The listing builds one solid part. Answer for the finished solid, in the listing's coordinates (mm). Face numbers are marked on the shaded views. A direction names the side the tool comes from. Round coordinates to 2 decimals unless told otherwise and drop trailing zeros. Order: outer loops, then holes, each group sorted by start corner. A loop starts at its lowest first (then second) coordinate and runs counter-clockwise, first axis right, second up. Notation, with made-up numbers: (29, 32.5) -> (38, 32.5) arc R18 cw to (38, 66.5) -> close; hole circle Ø10 at (47, 44.5). An arc over 180 degrees is marked (long way). Answer in a Markdown table with one row per item. Add a question column.
```python
from build123d import *

# Parameters (mm, degrees)
F0_R     = 1
F0_R_2   = 2.35
F1_DEPTH = 36
F2_W     = 98.13832
F2_H     = 30
F3_DEPTH = 26
F4_R     = 5
F5_SIZE  = 7
F7_DEPTH = 36


with BuildPart() as f1:
    # F0 (on Front) → F1 (new body)
    with BuildSketch(Plane.XZ):
        with BuildLine():
            Line((80, 15), (0, 15))
            ThreePointArc((0, 15), (-15, 0), (0, -15))
            Line((0, -15), (130, -15))
            Line((130, -15), (130, 15))
            Line((130, 15), (120, 15))
            Line((120, 15), (120, -5))
            Line((120, -5), (80, -5))
            Line((80, -5), (80, 15))
        make_face()
        with Locations((0, -10)):
            Circle(F0_R, mode=Mode.SUBTRACT)
        with Locations((75.3, -1)):
            Circle(F0_R_2, mode=Mode.SUBTRACT)
        with Locations((124.7, -1)):
            Circle(F0_R_2, mode=Mode.SUBTRACT)
        with Locations((-10, 0)):
            Circle(F0_R, mode=Mode.SUBTRACT)
        with Locations((10, 0)):
            Circle(F0_R, mode=Mode.SUBTRACT)
        with Locations((0, 10)):
            Circle(F0_R, mode=Mode.SUBTRACT)
        with Locations((75.3, 11)):
            Circle(F0_R_2, mode=Mode.SUBTRACT)
        with Locations((124.7, 11)):
            Circle(F0_R_2, mode=Mode.SUBTRACT)
    extrude(amount=F1_DEPTH)

    # F2 (on face) → F3 (cut)
    with BuildSketch(Plane(origin=(0, 0, 0), x_dir=(-1, 0, 0), z_dir=(0, 1, 0))):
        with Locations((-20.93084, 0)):
            Rectangle(F2_W, F2_H)
    extrude(amount=-F3_DEPTH, mode=Mode.SUBTRACT)

    # F4
    f4_edges = [f1.edges().sort_by_distance(p)[0] for p in [
        (80, -18, 15),
        (120, -18, 15),
    ]]
    fillet(f4_edges, radius=F4_R)

    # F5
    f5_edges = [f1.edges().sort_by_distance(p)[0] for p in [
        (130, -18, -15),
    ]]
    chamfer(f5_edges, length=F5_SIZE)

    # F6 (on face) → F7 (join)
    with BuildSketch(Plane.XZ.offset(36)):
        Polygon((119.393398, -18.606602), (123, -15), (115.786797, -15), align=None)
    extrude(amount=-F7_DEPTH)


solid = f1.part
```
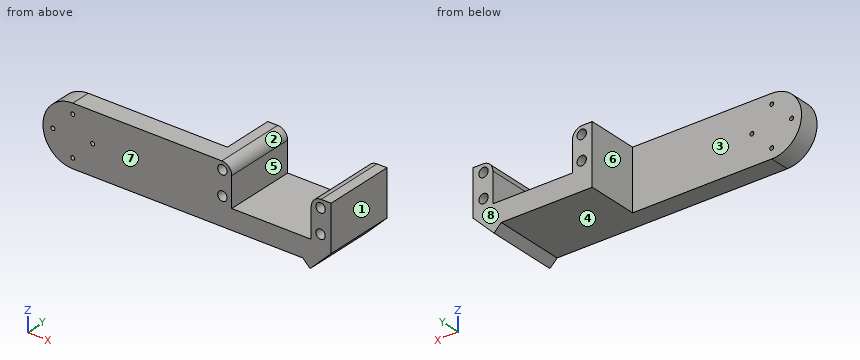
Item 1: For a pull along X with two mould halves and no side action, classify the marked faces 1, 2 and 3 as released by +X, released by -X, zero draft, split by the parting line, or undercut.
Item 2: Find the intervals of material crossed by probe 1 along Z at (x, y) = (75, -13); probe 2 along Z at (x, y) = (10, -33); probe 3 along X at (y, z) = (-6, 12.5), in increasing order. Write a range as [from, to].
Item 3: The part is cut by section A-A, the plane y = -11.5. Give the vertices of the cut face in (x, z).
Item 4: A tool of negligible diameter and unlimited length cuts with its end or side. For the marked faces 4, 5, 6, 7 and 8, from which of +Z, -Z, +X, -X, +Y, -Y can it reach the whole face along a straight path? Write none if from no direction.
Item 5: The part is cut by section B-B, the plane z = 5. Give the vertices of the cut face in (x, y), and give its area (3 significant figures).
Item 6: The part is cut by section D-D, the plane x = 87. Give the vertices of the cut face in (y, z), and give its area (3 significant figures).
Item 7: Flat-ended cylindrical pins translate along their axes: P1, Ø18, axis at x = 32, y = -25.5, coming from the -Z side; P2, Ø1.2, axis at x = 0, z = 10, coming from the -Y side; P3, Ø4, axis at x = 67, y = -25, coming from the +Z side; P4, Ø16.5, axis at y = -12, z = -0.5, coming from the -X side. Find the tip coordinate at first contact, or state that the pin passes through.
Item 8: The part is cut by section C-C, the plane x = 55. Give the vertices of the cut face in (y, z).
Resolved:
| question | item | result |
|---|---|---|
| 1 | face 1 | released by +X |
| 1 | face 2 | undercut |
| 1 | face 3 | zero draft |
| 2 | probe 1 | [-15, -3.33], [1.33, 8.67], [13.33, 15] |
| 2 | probe 2 | [-15, -1], [1, 15] |
| 2 | probe 3 | [70, 73.49], [77.11, 79.33], [120.67, 122.89], [126.51, 130] |
| 3 | outline | (70, -15) -> (115.79, -15) -> (119.39, -18.61) -> (130, -8) -> (130, 15) -> (125, 15) arc R5 ccw to (120, 10) -> (120, -5) -> (80, -5) -> (80, 10) arc R5 ccw to (75, 15) -> (70, 15) -> close; hole circle Ø4.7 at (75.3, -1); hole circle Ø4.7 at (75.3, 11); hole circle Ø4.7 at (124.7, -1); hole circle Ø4.7 at (124.7, 11) |
| 4 | face 4 | -Z, -X, +Y, -Y |
| 4 | face 5 | +Z, +Y, -Y |
| 4 | face 6 | +Z, -Z, -X, +Y |
| 4 | face 7 | +Z, -Z, +X, -X, -Y |
| 4 | face 8 | +Z, -Z, +X, -X, +Y |
| 5 | outline | (-14.14, -36) -> (80, -36) -> (80, 0) -> (70, 0) -> (70, -26) -> (-14.14, -26) -> close; (120, -36) -> (130, -36) -> (130, 0) -> (120, 0) -> close |
| 5 | area | 1,560 mm2 |
| 6 | outline | (-36, -15) -> (0, -15) -> (0, -5) -> (-36, -5) -> close |
| 6 | area | 360 mm2 |
| 7 | P1 | z = -15 |
| 7 | P2 | through |
| 7 | P3 | z = 15 |
| 7 | P4 | x = 70 |
| 8 | outline | (-36, -15) -> (-26, -15) -> (-26, 15) -> (-36, 15) -> close |
